Here's how the part is built. I have some questions about the finished solid (model axes, mm). Face numbers are marked on the shaded views. A direction names the side the tool comes from. Round coordinates to 2 decimals unless told otherwise and drop trailing zeros. Loops run counter-clockwise (first coordinate to the right, second up) from the corner with the lowest first, then second, coordinate; pieces in that order, holes last. Notation, with made-up numbers: (54, 61) -> (88, 61) arc R30 cw to (88, 86) -> close; hole circle Ø9 at (51.5, -21.5). An arc over 180 degrees is marked (long way). Use one line per item in the form item = value. Start each with the question number.
Item 1: If we section it at B-B (x = -1): Write out the boundary of the cut face in (y, z), then the cut area to 3 significant figures.
Item 2: If we section it at C-C (y = 2.5): Write out the boundary of the cut face in (x, z).
Item 3: I'm going to push flat-ended pins straight in: pin 1 Ø10.5 at (x, z) = (-1, 19.5) entering from +Y; pin 2 Ø4 at (x, z) = (0, -24) entering from -Y; pin 3 Ø4 at (x, y) = (-14, 13) entering from +Z; pin 4 Ø1 at (y, z) = (4, -8) entering from -X. Where does each tip first touch, or does it pass through?
Item 4: If we section it at D-D (y = 7.25): Write out the boundary of the cut face in (x, z), then the cut area to 3 significant figures.
Item 5: If I drill on L1, parallel to X at y = 11.75, z = 0; L2, parallel to Y at x = 10, z = 16.5; L3, parallel to X at y = 2.5, z = 24, over which ranges is the centre line in solid material (lowest first)? Write a range as [from, to].
Item 6: Thinking about a two-plate mould opening in Z: for the marked faces 4, 5 and 6, which applies, released by +Z, released by -Z, zero draft, split by the parting line, or undercut?
Item 7: For the marked faces 1, 2 and 3, which set-ups out of +Z, -Z, +X, -X, +Y, -Y let a thin tool reach every point of the face, with its end or its side?
Item 8: If we section it at A-A (z = 0): Write out the boundary of the cut face in (x, y), then the cut area to 3 significant figures.
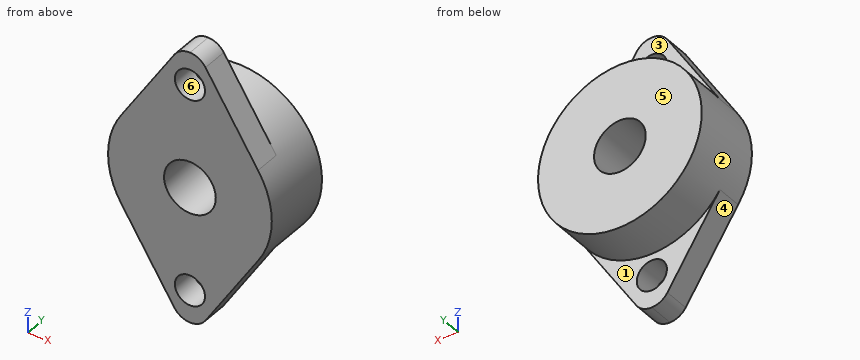
```python
from build123d import *

# Parameters (mm, degrees)
SKETCH1_R           = 19
BOSS_EXTRUDE1_DEPTH = 16.5
BOSS_EXTRUDE2_DEPTH = 6
SKETCH3_R           = 6
CUT_EXTRUDE1_DEPTH  = 41.317490001
SKETCH4_R           = 3.5
CUT_EXTRUDE2_DEPTH  = 39.255718527


with BuildPart() as part:
    # Sketch1 → Boss-Extrude1 (new body)
    with BuildSketch(Plane(origin=(0, 0, 0), x_dir=(1, 0, 0), z_dir=(0, 1, 0))):
        with Locations(Location((0, 0, 0), (0, 0, 270))):
            Circle(SKETCH1_R)
    extrude(amount=BOSS_EXTRUDE1_DEPTH)

    # Sketch2 → Boss-Extrude2 (add)
    with BuildSketch(Plane(origin=(0, 0, 0), x_dir=(1, 0, 0), z_dir=(0, 1, 0))):
        with BuildLine():
            Line((0, 10.549840688), (0, 22.89723562))
            ThreePointArc((0, 22.89723562), (-3.774822907, 25.136434317), (-3.61947725, 29.522681746))
            Line((-3.61947725, 29.522681746), (-15.801925878, 10.549840688))
            Line((-15.801925878, 10.549840688), (0, 10.549840688))
        make_face()
        with BuildLine():
            ThreePointArc((4.30138219, 27.19861781), (3.041536515, 24.157081295), (0, 22.89723562))
            Line((0, 22.89723562), (0, 10.549840688))
            Line((0, 10.549840688), (15.801925878, 10.549840688))
            Line((15.801925878, 10.549840688), (3.61947725, 29.522681746))
            ThreePointArc((3.61947725, 29.522681746), (4.127386808, 28.409636753), (4.30138219, 27.19861781))
        make_face()
        with BuildLine():
            ThreePointArc((3.61947725, 29.522681746), (2.062183493, 30.973440718), (0, 31.5))
            Line((0, 31.5), (0, 22.89723562))
            ThreePointArc((0, 22.89723562), (3.041536515, 24.157081295), (4.30138219, 27.19861781))
            ThreePointArc((4.30138219, 27.19861781), (4.127386808, 28.409636753), (3.61947725, 29.522681746))
        make_face()
        with BuildLine():
            Line((0, 22.89723562), (0, 31.5))
            ThreePointArc((0, 31.5), (-2.062183493, 30.973440718), (-3.61947725, 29.522681746))
            ThreePointArc((-3.61947725, 29.522681746), (-3.774822907, 25.136434317), (0, 22.89723562))
        make_face()
    boss_extrude2 = extrude(amount=BOSS_EXTRUDE2_DEPTH)

    # Sketch3 → Cut-Extrude1 (cut, through all)
    with BuildSketch(Plane(origin=(0, 16.5, 0), x_dir=(1, 0, 0), z_dir=(0, 1, 0))):
        with Locations(Location((0, 0, 0), (0, 0, 270))):
            Circle(SKETCH3_R)
    extrude(amount=-CUT_EXTRUDE1_DEPTH, mode=Mode.SUBTRACT)

    # Sketch4 → Cut-Extrude2 (cut, through all)
    with BuildSketch(Plane(origin=(0, 6, 0), x_dir=(1, 0, 0), z_dir=(0, 1, 0))):
        with Locations(Location((0, 24, 0), (0, 0, 270))):
            Circle(SKETCH4_R)
    cut_extrude2 = extrude(amount=-CUT_EXTRUDE2_DEPTH, mode=Mode.SUBTRACT)

    # Mirror1: Boss-Extrude2, Cut-Extrude2 across plane
    add(boss_extrude2.mirror(Plane.XY))
    add(cut_extrude2.mirror(Plane.XY), mode=Mode.SUBTRACT)


solid = part.part
```
Values found:
q1.outline = (0, -31.38) -> (6, -31.38) -> (6, -27.35) -> (0, -27.35) -> close; (0, -20.65) -> (6, -20.65) -> (6, -18.97) -> (16.5, -18.97) -> (16.5, -5.92) -> (0, -5.92) -> close; (0, 5.92) -> (16.5, 5.92) -> (16.5, 18.97) -> (6, 18.97) -> (6, 20.65) -> (0, 20.65) -> close; (0, 27.35) -> (6, 27.35) -> (6, 31.38) -> (0, 31.38) -> close
q1.area = 499 mm2
q2.outline = (-15.8, -10.55) -> (-3.62, -29.52) arc R4.3 ccw to (3.62, -29.52) -> (15.8, -10.55) arc R19 ccw to (15.8, 10.55) -> (3.62, 29.52) arc R4.3 ccw to (-3.62, 29.52) -> (-15.8, 10.55) arc R19 ccw to start; hole circle Ø12 at (0, 0); hole circle Ø7 at (0, -24); hole circle Ø7 at (0, 24)
q3.pin_1 = 16.5
q3.pin_2 = through
q3.pin_3 = 14.73
q3.pin_4 = -17.46
q4.outline = circle Ø38 at (0, 0); hole circle Ø12 at (0, 0)
q4.area = 1,020 mm2
q5.L1 = [-19, -6], [6, 19]
q5.L2 = [0, 6]
q5.L3 = [-7.17, -3.5], [3.5, 7.17]
q6.face_4 = released by -Z
q6.face_5 = zero draft
q6.face_6 = undercut
q7.face_1 = -Z, +Y
q7.face_2 = +Y
q7.face_3 = +Z, +Y
q8.outline = (-19, 0) -> (-6, 0) -> (-6, 16.5) -> (-19, 16.5) -> close; (6, 0) -> (19, 0) -> (19, 16.5) -> (6, 16.5) -> close
q8.area = 429 mm2
